Verification items for the finished model (mm, model axes). A direction names the side the tool comes from. Coordinates: 2 decimals unless noted, no trailing zeros. Use CSV: the item, a comma, the result in double quotes.
```python
from build123d import *

# Parameters (mm, degrees)
POCKET_DEPTH    = 5
SKETCH005_R     = 2.917562
POCKET001_DEPTH = 20.6489723154
SKETCH006_R     = 2.917562
POCKET002_DEPTH = 23.0482544438
SKETCH007_R     = 3
POCKET003_DEPTH = 24.5764305412


with BuildPart() as part:
    # Sketch002 → Loft section 0
    with BuildSketch(Plane.XY.offset(10)):
        with BuildLine():
            ThreePointArc((-11.343506, 11.1193269091), (-20.3555434545, 2.1072894545), (-11.343506, -6.904748))
            Line((-11.343506, -6.904748), (18.7414073452, -6.904748))
            ThreePointArc((18.7414073452, -6.904748), (27.7534447997, 2.1072894545), (18.7414073452, 11.1193269091))
            Line((-11.343506, 11.1193269091), (18.7414073452, 11.1193269091))
        make_face()
    # Sketch003 → Loft section 1
    with BuildSketch(Plane.XY):
        with BuildLine():
            ThreePointArc((-12.0831570349, 16.0971179095), (-26.0729854896, 2.1072894547), (-12.0831570349, -11.882539))
            Line((-12.0831570349, -11.882539), (24.0627546777, -11.882539))
            ThreePointArc((24.0627546777, -11.882539), (38.0525831324, 2.1072894547), (24.0627546777, 16.0971179095))
            Line((-12.0831570349, 16.0971179095), (24.0627546777, 16.0971179095))
        make_face()
    loft()

    # Sketch001 → Pocket (cut)
    with BuildSketch(Plane.XY.offset(10)):
        Polygon((-6.094202, 5.983397), (-6.094202, 8.088668), (11.634386, 7.313041), (13.752719, 6.511327), (13.97268, -0.847062), (13.185631, -1.329644), (-3.545716, -5.318575), (-4.282123, -4.272569), (-6.45014, 0.995308), align=None)
    extrude(amount=-POCKET_DEPTH, mode=Mode.SUBTRACT)

    # Sketch005 → Pocket001 (cut, through all)
    with BuildSketch(Plane(origin=(-6.4881258553, 0.462977012, 0), x_dir=(0.0711766059, 0.9974637291, 0), z_dir=(0.9974637291, -0.0711766059, 0))):
        with Locations((4.141323, 8.428433)):
            Circle(SKETCH005_R)
    extrude(amount=-POCKET001_DEPTH, mode=Mode.SUBTRACT)

    # Sketch006 → Pocket002 (cut, through all)
    with BuildSketch(Plane(origin=(-5.1655859853, -2.1259187014, 0), x_dir=(-0.3805833694, 0.9247466134, 0), z_dir=(0.9247466134, 0.3805833694, 0))):
        with Locations((0.622215, 8.350686)):
            Circle(SKETCH006_R)
    extrude(amount=-POCKET002_DEPTH, mode=Mode.SUBTRACT)

    # Sketch007 → Pocket003 (cut, through all)
    with BuildSketch(Plane(origin=(13.9349074201, 0.4165498958, 0), x_dir=(0.029879202, -0.999553517, 0), z_dir=(-0.999553517, -0.029879202, 0))):
        with Locations((-2.85774, 8.49941)):
            Circle(SKETCH007_R)
    extrude(amount=-POCKET003_DEPTH, mode=Mode.SUBTRACT)


solid = part.part
```
1) Mould release check, pull along X, two halves, no side actions. Record for faces 4 (the flat face through (-5.2, -2.04, 5.29)), 5 (the flat face through (4, 3, 5)), 6 (the flat face through (-15, 0, 10)): released by +X, released by -X, zero draft, split by the parting line, or undercut.
Return value:
face 4,"undercut"
face 5,"undercut"
face 6,"zero draft"
2) Scan lines: L1, parallel to Y at x = -9, z = 7.75; L2, parallel to Z at x = 13, y = 2.5; L3, parallel to Y at x = 18, z = 6.75. Record each from-to range of solid material in increasing order.
Return value:
L1,"-8.02 to -6.12, 0.06 to 1.95, 7.64 to 12.24"
L2,"0 to 5"
L3,"-8.52 to 0.96, 5.84 to 12.74"
3) Gauge pin test, flat ends, axial feed: pin 1 (1.7 mm diameter, centred on y = 7, z = 7, fed in from +X); pin 2 (3 mm diameter, centred on x = 7.5, z = 8, fed in from -Y); pin 3 (4 mm diameter, centred on x = 1.5, y = 4.5, fed in from +Z). Record the tip position at first contact, or that the pin passes through.
Return value:
pin 1,"x = 30.65"
pin 2,"y = -8.65"
pin 3,"z = 5"
4) Set-up check for faces 1 (the cylindrical face through (22.9, 3.6, 5.5)), 2 (the flat face through (4, 9, 10)), 3 (the flat face through (12.679, 6.918, 7.535)): record each of +Z, -Z, +X, -X, +Y, -Y from which the full face is reachable in a straight line by a thin tool's end or side.
Return value:
face 1,"none"
face 2,"+Z, +X, -X, +Y, -Y"
face 3,"+Z"
